Autodesk Inventor part; units mm, degrees
ref_plane "Work Plane4" through (7.6, 2, 20) normal (-1, 0, 0) x (0, 0, 1)
ref_plane "YZ Plane" through (0, 0, 0) normal (1, 0, 0) x (0, 1, 0)
ref_plane "XZ Plane" through (0, 0, 0) normal (0, 1, 0) x (-1, 0, 0)
sketch "Sketch1" plane through (0, 0, 0) normal (0, 0, 1) x (1, 0, 0)
  line L0 (0, 0) -> (15.2, 0)
  line L1 (15.2, 0) -> (15.2, 12)
  line L2 (15.2, 12) -> (0, 12)
  line L3 (0, 12) -> (0, 0)
  line L4 (1.6, 10) -> (13.6, 10)
  line L5 (13.6, 10) -> (13.6, 2)
  line L6 (13.6, 2) -> (1.6, 2)
  line L7 (1.6, 2) -> (1.6, 10)
  dimension "d0" = 15.2
  dimension "d1" = 12
  dimension "d2" = 1.6
  dimension "d3" = 2
  dimension "d4" = 2
  dimension "d5" = 1.6
extrude "Extrusion1" add sketch "Sketch1" along normal blind 20
sketch "Sketch2" plane through (0, 0, 0) normal (1, 0, 0) x (0, 1, 0)
  line L0 (0, 0) -> (12, 0) construction
  line L1 (6, 13.0663) -> (6, -2.0093) construction
  line L2 (0, 0) -> (0, 20) construction
  line L3 (12, 0) -> (12, 20) construction
  line L4 (6, 0) -> (12, 3.8224)
  line L5 (12, 3.8224) -> (12, 0)
  line L6 (12, 0) -> (6, 0)
  dimension "d8" = 12
  dimension "d9" = 6
  dimension "d10" = 32.5
extrude "Extrusion2" cut sketch "Sketch2" along normal through all
sketch "Sketch9" plane through (0, 0, 20) normal (-1, 0, 0) x (0, 0, 1)
  line L0 (-20, 0) -> (0, 0) construction
  line L1 (0, 12) -> (0, 0) construction
  line L2 (-16.1776, 12) -> (0, 12) construction
  line L3 (-20, 0) -> (-20, 14.5103) construction
  line L4 (-20, 0) -> (0, 0)
  line L5 (0, 12) -> (0, 0)
  line L6 (0, 12) -> (-20, 12)
  arc A0 (-20, 12) -> (-20, 0) centre (-20, 6) ccw
extrude "Extrusion8" add sketch "Sketch9" along normal blind 2.4
sketch "Sketch4" plane through (1.6, 2, 20) normal (1, 0, 0) x (0, 0, -1)
  circle A0 centre (20, 4) radius 3
  point P0 (20, -2)
  dimension "d14" = 6
extrude "Extrusion3" cut sketch "Sketch4" along normal through all both and the other way through all
sketch "Sketch11" plane through (15.2, 12, 20) normal (0, 1, 0) x (1, 0, 0)
  line L0 (0, 0) -> (-17.6, 0) construction
  line L1 (-15.2, 26) -> (-15.2, 20) construction
  line L2 (-15.2, 26) -> (-16, 26)
  line L3 (-16, 26) -> (-16, 10)
  line L4 (-16, 10) -> (-15.2, 10)
  line L5 (-15.2, 10) -> (-15.2, 26)
  line L6 (-15.2, 20) -> (-13.6, 20) construction
  dimension "d38" = 10
  dimension "d39" = 0.8
extrude "Extrusion9" cut sketch "Sketch11" against normal through all
ref_plane "Work Plane4" through (7.6, 2, 20) normal (-1, 0, 0) x (0, 0, 1)
mirror "Mirror3" about plane through (7.6, 2, 20) normal (-1, 0, 0) of "Extrusion8", "Extrusion3", "Extrusion9"
sketch "Sketch17" plane through (-2.4, 0, 20) normal (-1, 0, 0) x (0, 0, 1)
  circle A0 centre (-20, 6) radius 3
  line L0 (0, 0) -> (0, 12) construction
  arc A1 (-20, 12) -> (-20, 0) centre (-20, 6) ccw construction
  line L1 (5, -10.5) -> (-28, -10.5)
  line L2 (-28, -10.5) -> (-28, 22.5)
  line L3 (-28, 22.5) -> (5, 22.5)
  line L4 (5, 22.5) -> (5, -10.5)
  line L5 (-20, 6) -> (17.487, 6) construction
  circle A2 centre (-23, 17.5) radius 2.2
  circle A3 centre (0, 17.5) radius 2.2
  circle A4 centre (-23, -5.5) radius 2.2
  circle A5 centre (0, -5.5) radius 2.2
  dimension "d82" = 33
  dimension "d83" = 5
  dimension "d84" = 16.5
  dimension "d85" = 4.4
  dimension "d86" = 5
  dimension "d87" = 5
  dimension "d90" = 23
  dimension "d93" = 23
extrude "Extrusion15" add sketch "Sketch17" along normal blind 3
equation "\"d9\" = 0.5 * d8"
equation "\"d84\" = 0.5 * d82"
properties part number "chain_end_extruder-back"
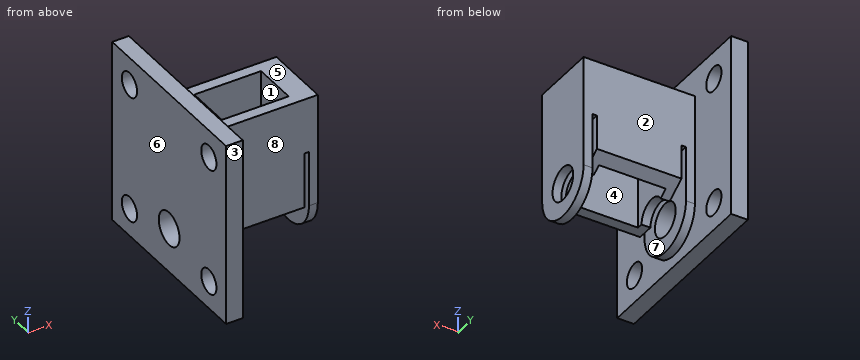
Geometry check sheet. Reference: the model listing, model coordinates, mm. Face numbers are marked on the shaded views. A direction names the side the tool comes from. Coordinates: 2 decimals unless noted, no trailing zeros. Order: outer loops, then holes, each group sorted by start corner. A loop starts at its lowest first (then second) coordinate and runs counter-clockwise, first axis right, second up.
Q1. Thickness scan on probe 1 along X at (y, z) = (8.5, 9.5); probe 2 along Y at (x, z) = (-3.7, 20); probe 3 along X at (y, z) = (9, 15). Record the ranges inside material, lowest first.
Reply:
probe 1: x = -5.4 to -0.8, 0 to 1.6, 13.6 to 15.2, 16 to 17.6
probe 2: y = -10.5 to -7.7, -3.3 to 15.3, 19.7 to 22.5
probe 3: x = -5.4 to 1.6, 13.6 to 17.6
Q2. Sectioned sample at B-B on x = 11.25. Record the cut outline in (y, z), and give its area (3 significant figures).
Reply:
outline: (0, 0) - (2, 0) - (2, 20) - (0, 20) - close; (10, 2.55) - (12, 3.82) - (12, 20) - (10, 20) - close
area: 73.6 mm2
Q3. Sectioned sample at C-C on y = 17.5. Record the cut outline in (x, z).
Reply:
outline: (-5.4, -8) - (-2.4, -8) - (-2.4, -5.2) - (-5.4, -5.2) - close; (-5.4, -0.8) - (-2.4, -0.8) - (-2.4, 17.8) - (-5.4, 17.8) - close; (-5.4, 22.2) - (-2.4, 22.2) - (-2.4, 25) - (-5.4, 25) - close
Q4. Draft check along Y on the marked faces 1, 2 and 3. Enter one of: released by +Y, released by -Y, zero draft, split by the parting line, or undercut.
Reply:
face 1: undercut
face 2: released by +Y
face 3: released by -Y
Q5. Sectioned sample at D-D on y = 6. Record the cut outline in (x, z), and give its area (3 significant figures).
Reply:
outline: (-5.4, -8) - (-2.4, -8) - (-2.4, -6) - (-0.8, -6) - (-0.8, -3) - (-5.4, -3) - close; (-5.4, 3) - (-0.8, 3) - (-0.8, 10) - (0, 10) - (0, 3) - (1.6, 3) - (1.6, 20) - (-2.4, 20) - (-2.4, 25) - (-5.4, 25) - close; (13.6, 3) - (15.2, 3) - (15.2, 10) - (16, 10) - (16, 3) - (17.6, 3) - (17.6, 20) - (13.6, 20) - close; (16, -6) - (17.6, -6) - (17.6, -3) - (16, -3) - close
area: 215 mm2
Q6. Tool access check on the marked faces 4, 5, 6, 7 and 8. Record the directions out of +Z, -Z, +X, -X, +Y, -Y that give a thin tool (end or side, any length) a straight path to the whole face; none if there is none.
Reply:
face 4: +Z, -Z
face 5: +Z, +X, +Y, -Y
face 6: +Z, -Z, -X, +Y, -Y
face 7: -Z, +Y, -Y
face 8: +Z, -Z, +X, -Y
Q7. Sectioned sample at A-A on z = 8.5. Record the cut outline in (x, y), and give its area (3 significant figures).
Reply:
outline: (-5.4, -10.5) - (-2.4, -10.5) - (-2.4, 0) - (-0.8, 0) - (-0.8, 12) - (-2.4, 12) - (-2.4, 22.5) - (-5.4, 22.5) - close; (0, 0) - (15.2, 0) - (15.2, 12) - (0, 12) - close; (16, 0) - (17.6, 0) - (17.6, 12) - (16, 12) - close; hole (1.6, 2) - (13.6, 2) - (13.6, 10) - (1.6, 10) - close
area: 224 mm2
Q8. Depth check by flat-ended pin: pin 1 Ø2.5 at (y, z) = (-5.5, 20) entering from +X; pin 2 Ø2 at (y, z) = (16, 8) entering from +X; pin 3 Ø1.5 at (x, z) = (11.5, 18) entering from -Y; pin 4 Ø0.9 at (x, y) = (16, 6.5) entering from -Z. Enter the tip coordinate at first touch or a pass-through.
Reply:
pin 1: passes through
pin 2: stops at x = -2.4
pin 3: stops at y = 0
pin 4: stops at z = -6
